The model under review builds one solid part; all positions refer to its coordinate system, in mm. Face numbers are marked on the shaded views. A direction names the side the tool comes from. Give positions to 0.01 mm unless a question says otherwise; leave off trailing zeros. Order: outer loops, then holes, each group sorted by start corner. A loop starts at its lowest first (then second) coordinate and runs counter-clockwise, first axis right, second up. Notation, with made-up numbers: (-31, -28) - (2, -28) arc R28 ccw to (2, 7) - close; hole circle Ø10 at (64, -3). An arc over 180 degrees is marked (long way). Use a Markdown table: item, result. Add a question column.
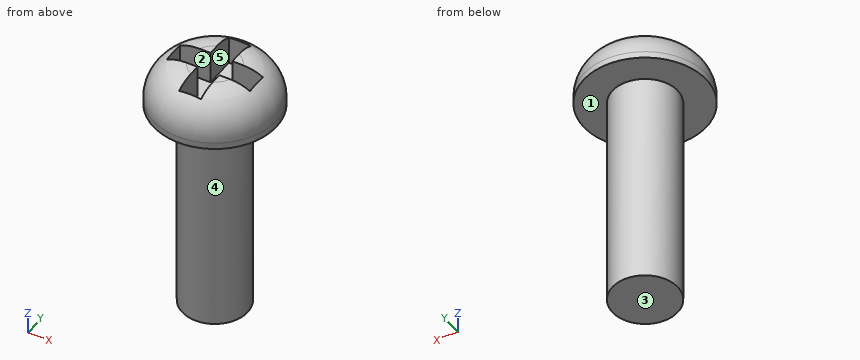
Autodesk Inventor part; units mm, degrees
ref_plane "YZ Plane" through (0, 0, 0) normal (1, 0, 0) x (0, 1, 0)
ref_plane "XZ Plane" through (0, 0, 0) normal (0, 1, 0) x (-1, 0, 0)
ref_plane "XY Plane" through (0, 0, 0) normal (0, 0, 1) x (1, 0, 0)
sketch "Эскиз1" plane through (0, 0, 0) normal (0, 0, 1) x (1, 0, 0)
  circle A0 centre (-4.8391, -17.7214) radius 1.5
  point P0 (0, 0)
extrude "Выдавливание1" add sketch "Эскиз1" against normal blind 10
sketch "Эскиз2" plane through (-4.8391, -17.7214, 0) normal (0, 0, 1) x (1, 0, 0)
  circle A0 centre (0, 0) radius 2.816
  point P0 (4.8391, 17.7214)
extrude "Выдавливание2" add sketch "Эскиз2" along normal blind 2
fillet "Сопряжение1" radius 1.7 1 edges at (-7.6551, -17.7214, 2)
sketch "Эскиз3" plane through (-4.8391, -17.7214, 2) normal (0, 0, 1) x (1, 0, 0)
  line L0 (-0.5, -1.9) -> (0.5, -1.9)
  line L1 (0.5, 1.9) -> (-0.5, 1.9)
  line L2 (1.9, -0.5) -> (1.9, 0.5)
  line L3 (-1.9, 0.5) -> (-1.9, -0.5)
  line L4 (-0.5, 1.9) -> (-0.5, 0.5)
  line L5 (-0.5, -0.5) -> (-0.5, -1.9)
  line L6 (1.9, 0.5) -> (0.5, 0.5)
  line L7 (-0.5, 0.5) -> (-1.9, 0.5)
  line L8 (0.5, -1.9) -> (0.5, -0.5)
  line L9 (0.5, 0.5) -> (0.5, 1.9)
  line L10 (-1.9, -0.5) -> (-0.5, -0.5)
  line L11 (0.5, -0.5) -> (1.9, -0.5)
  point P0 (4.8391, 17.7214)
  point P1 (0, 0)
extrude "Выдавливание3" cut sketch "Эскиз3" against normal blind 1.5
thread "Резьба1"
properties part number "Винт М3х10"
Q1. Machinability: for the marked faces 1 and 2, which of the approach directions +Z, -Z, +X, -X, +Y, -Y give a long, thin tool a straight path to every point of the face, cutting with its end or side? Answer none if there is none.
Q2. We need section A-A (z = -1). Write out the cut boundary in (x, y), plus the area to 3 significant figures.
Q3. Draft analysis for pull direction X (two halves, no side actions). For the marked faces 3, 4 and 5, state which applies: pulls with the +X half, pulls with the -X half, needs draft (parallel to the pull), parting line crosses it, or undercut.
Q4. Wall thickness on probe 1 along X at (y, z) = (-19.1, 1.75); probe 2 along Z at (x, y) = (-4.85, -17.3); probe 3 along X at (y, z) = (-18.9, -2.25): over which ranges is each line inside the solid? List them lowest first.
Q5. Clearance check with flat-ended pins moving along their axes: P1, Ø0.5, axis at x = -5, z = 1, coming from the +Y side; P2, Ø1.1, axis at x = -5, z = 1.5, coming from the -Y side (3 decimals); P3, Ø0.5, axis at y = -17.5, z = 1.5, coming from the -X side. State where each tip first meets the part, or that it passes through.
Here are the results:
| question | item | result |
|---|---|---|
| 1 | face 1 | -Z |
| 1 | face 2 | +Z |
| 2 | outline | circle Ø3 at (-4.84, -17.72) |
| 2 | area | 7.07 mm2 |
| 3 | face 3 | needs draft |
| 3 | face 4 | parting line crosses it |
| 3 | face 5 | undercut |
| 4 | probe 1 | -6.29 to -5.34, -4.34 to -3.39 |
| 4 | probe 2 | -10 to 0.5 |
| 4 | probe 3 | -5.77 to -3.91 |
| 5 | P1 | y = -14.97 |
| 5 | P2 | y = -20.405 |
| 5 | P3 | x = -7.36 |
